Autodesk Inventor part; units mm, degrees
ref_plane "YZ Plane" through (0, 0, 0) normal (1, 0, 0) x (0, 1, 0)
ref_plane "XZ Plane" through (0, 0, 0) normal (0, 1, 0) x (-1, 0, 0)
ref_plane "XY Plane" through (0, 0, 0) normal (0, 0, 1) x (1, 0, 0)
sketch "Sketch1" plane through (0, 0, 0) normal (0, 1, 0) x (-1, 0, 0)
  line L0 (-38.1, -50.8) -> (38.1, -50.8)
  line L1 (38.1, -50.8) -> (38.1, 50.8)
  line L2 (38.1, 50.8) -> (-38.1, 50.8)
  line L3 (-38.1, 50.8) -> (-38.1, -50.8)
  line L4 (-38.1, -50.8) -> (38.1, 50.8) construction
  line L5 (38.1, -50.8) -> (-38.1, 50.8) construction
  point P0 (0, 0)
  dimension "d0" = 101.6
  dimension "d1" = 76.2
extrude "Extrusion1" add sketch "Sketch1" along normal blind 3.175
sketch "Sketch2" plane through (0, 3.175, 0) normal (0, 1, 0) x (1, 0, 0)
  line L0 (-9.9878, -31.7793) -> (-30.8713, -31.7793) construction
  line L1 (-9.9878, -30.7915) -> (-30.8713, -30.7915)
  line L2 (-30.8713, -32.7672) -> (-9.9878, -32.7672)
  arc A0 (-9.9878, -32.7672) -> (-9.9878, -30.7915) centre (-9.9878, -31.7793) ccw
  arc A1 (-30.8713, -30.7915) -> (-30.8713, -32.7672) centre (-30.8713, -31.7793) ccw
  line L3 (7.9124, -32.7672) -> (32.6873, -32.7672) construction
  line L4 (7.9124, -33.755) -> (32.6873, -33.755)
  line L5 (32.6873, -31.7793) -> (7.9124, -31.7793)
  arc A2 (7.9124, -31.7793) -> (7.9124, -33.755) centre (7.9124, -32.7672) ccw
  arc A3 (32.6873, -33.755) -> (32.6873, -31.7793) centre (32.6873, -32.7672) ccw
  line L6 (20.2998, -22.4401) -> (12.582, -22.4401) construction
  line L7 (20.2998, -21.5321) -> (12.582, -21.5321)
  line L8 (12.582, -23.3481) -> (20.2998, -23.3481)
  arc A4 (20.2998, -23.3481) -> (20.2998, -21.5321) centre (20.2998, -22.4401) ccw
  arc A5 (12.582, -21.5321) -> (12.582, -23.3481) centre (12.582, -22.4401) ccw
  line L9 (20.2998, -13.3603) -> (4.4102, -13.3603) construction
  line L10 (20.2998, -12.2445) -> (4.4102, -12.2445)
  line L11 (4.4102, -14.4761) -> (20.2998, -14.4761)
  arc A6 (20.2998, -14.4761) -> (20.2998, -12.2445) centre (20.2998, -13.3603) ccw
  arc A7 (4.4102, -12.2445) -> (4.4102, -14.4761) centre (4.4102, -13.3603) ccw
  line L12 (-9.9878, 31.7793) -> (-30.8713, 31.7793) construction
  line L13 (-9.9878, 30.7915) -> (-30.8713, 30.7915)
  line L14 (-30.8713, 32.7672) -> (-9.9878, 32.7672)
  arc A8 (-9.9878, 30.7915) -> (-9.9878, 32.7672) centre (-9.9878, 31.7793) ccw
  arc A9 (-30.8713, 32.7672) -> (-30.8713, 30.7915) centre (-30.8713, 31.7793) ccw
  line L15 (7.9124, 32.7672) -> (32.6873, 32.7672) construction
  line L16 (7.9124, 33.755) -> (32.6873, 33.755)
  line L17 (32.6873, 31.7793) -> (7.9124, 31.7793)
  arc A10 (7.9124, 33.755) -> (7.9124, 31.7793) centre (7.9124, 32.7672) ccw
  arc A11 (32.6873, 31.7793) -> (32.6873, 33.755) centre (32.6873, 32.7672) ccw
  line L18 (20.2998, 22.4401) -> (12.582, 22.4401) construction
  line L19 (20.2998, 21.5321) -> (12.582, 21.5321)
  line L20 (12.582, 23.3481) -> (20.2998, 23.3481)
  arc A12 (20.2998, 21.5321) -> (20.2998, 23.3481) centre (20.2998, 22.4401) ccw
  arc A13 (12.582, 23.3481) -> (12.582, 21.5321) centre (12.582, 22.4401) ccw
  line L21 (20.2998, 13.3603) -> (4.4102, 13.3603) construction
  line L22 (20.2998, 12.2445) -> (4.4102, 12.2445)
  line L23 (4.4102, 14.4761) -> (20.2998, 14.4761)
  arc A14 (20.2998, 12.2445) -> (20.2998, 14.4761) centre (20.2998, 13.3603) ccw
  arc A15 (4.4102, 14.4761) -> (4.4102, 12.2445) centre (4.4102, 13.3603) ccw
  point P0 (-20.4296, -31.7793)
  point P1 (20.2998, -32.7672)
  point P2 (16.4409, -22.4401)
  point P3 (12.355, -13.3603)
  point P4 (0, -25.2547)
  point P5 (-20.4296, 31.7793)
  point P6 (20.2998, 32.7672)
  point P7 (16.4409, 22.4401)
  point P8 (12.355, 13.3603)
extrude "Extrusion2" cut sketch "Sketch2" against normal blind 3.175
properties part number "top frame 4x4" material "Nickel-Copper Alloy 400"
Check sheet for the modelled part. Datum: model origin and axes. Units: mm. A direction names the side the tool comes from. Round coordinates to 2 decimals unless told otherwise and drop trailing zeros. Loops run counter-clockwise (first coordinate to the right, second up) from the corner with the lowest first, then second, coordinate; pieces in that order, holes last. Notation, with made-up numbers: (-39.5, 45) -> (9.5, 45) arc R19 ccw to (9.5, 58) -> close; hole circle Ø4 at (61, 44). An arc over 180 degrees is marked (long way). Write item = value, one per line. Start each with the question number.
1) Set-up check for faces 1 (the flat face through (20, 2, 33.755)), 2 (the flat face through (1, 3.175, 1)): record each of +Z, -Z, +X, -X, +Y, -Y from which the full face is reachable in a straight line by a thin tool's end or side.
2) Sectioned sample at B-B, the plane y = 1.7. State how many separate pieces and enclosed holes the cut face has, plus the area to 3 significant figures.
3) Release check for a two-part mould opening along Z. For faces 3 (the flat face through (-21, 2, -32.767)), 4 (the flat face through (1, 2, -50.8)), 5 (the flat face through (38.1, 2, 1)) record: released by +Z, released by -Z, zero draft, split by the parting line, or undercut.
4) Sectioned sample at A-A, the plane x = -13. Record the cut outline in (y, z) (1 decimal).
5) Thickness scan on probe 1 along Z at (x, y) = (-15.5, 2.35); probe 2 along Z at (x, y) = (23.5, 2.75) (3 decimals); probe 3 along Z at (x, y) = (9, 0.55) (1 decimal). Record the ranges inside material, lowest first.
Results are:
q1.face_1 = +Y, -Y
q1.face_2 = +Z, -Z, +X, -X, +Y
q2.separate_pieces = 1
q2.enclosed_holes = 8
q2.area = 7,440 mm^2
q3.face_3 = undercut
q3.face_4 = released by -Z
q3.face_5 = zero draft
q4.outline = (0, -50.8) -> (3.2, -50.8) -> (3.2, -32.8) -> (0, -32.8) -> close; (0, -30.8) -> (3.2, -30.8) -> (3.2, 30.8) -> (0, 30.8) -> close; (0, 32.8) -> (3.2, 32.8) -> (3.2, 50.8) -> (0, 50.8) -> close
q5.probe_1 = -50.8 to -32.77, -30.79 to 30.79, 32.77 to 50.8
q5.probe_2 = -50.8 to -33.755, -31.779 to 31.779, 33.755 to 50.8
q5.probe_3 = -50.8 to -33.8, -31.8 to -14.5, -12.2 to 12.2, 14.5 to 31.8, 33.8 to 50.8
